```python
from build123d import *

# Parameters (mm, degrees)
SALIENTE_EXTRUIR1_DEPTH = 5


with BuildPart() as part:
    # Croquis1 → Saliente-Extruir1 (new, symmetric)
    with BuildSketch(Plane(origin=(0, 0, 0), x_dir=(-1, 0, 0), z_dir=(0, 1, 0))):
        with BuildLine():
            Line((34.242733527, 21.931170499), (171.411434738, 32.390487311))
            ThreePointArc((171.411434738, 32.390487311), (200.969948773, 5.053051121), (171.517245245, -22.398350016))
            Line((171.517245245, -22.398350016), (-0.718901979, -9.934021338))
            ThreePointArc((-0.718901979, -9.934021338), (-9.877207042, -1.281554151), (-3.23027027, 9.421621622))
            Line((-3.23027027, 9.421621622), (31.76972973, 21.421621622))
            ThreePointArc((31.76972973, 21.421621622), (32.99001932, 21.755079583), (34.242733527, 21.931170499))
        make_face()
        with BuildLine():
            Line((-0.574544152, -7.939237937), (171.661603072, -20.403566614))
            ThreePointArc((171.661603072, -20.403566614), (198.969952502, 5.049188644), (171.563496279, 30.396276368))
            Line((171.563496279, 30.396276368), (34.394795068, 19.936959556))
            ThreePointArc((34.394795068, 19.936959556), (33.393629898, 19.796228261), (32.418378378, 19.52972973))
            Line((32.418378378, 19.52972973), (-2.581621622, 7.52972973))
            ThreePointArc((-2.581621622, 7.52972973), (-7.893832134, -1.02421396), (-0.574544152, -7.939237937))
        make_face(mode=Mode.SUBTRACT)
    extrude(amount=SALIENTE_EXTRUIR1_DEPTH, both=True)


solid = part.part
```
Verification items for the finished model (mm, model axes). A direction names the side the tool comes from. Give positions to 0.01 mm unless a question says otherwise; leave off trailing zeros. Order: outer loops, then holes, each group sorted by start corner. A loop starts at its lowest first (then second) coordinate and runs counter-clockwise, first axis right, second up. Notation, with made-up numbers: M 33.25,65.25 L 61.25,65.25 A19 ccw 61.25,79.25 Z; hole C 62.25,18 d9. An arc over 180 degrees is marked long. Answer in a Markdown table with one row per item. Add a question column.
Item 1: Mould release check, pull along Z, two halves, no side actions. Record for faces 1 (the cylindrical face through (-200.96, 0.07, 5.69)), 2 (the flat face through (-101.867, 0.07, 27.088)), 3 (the cylindrical face through (-198.964, 0.07, 4.463)): released by +Z, released by -Z, zero draft, split by the parting line, or undercut.
Item 2: Section check C-C, the plane z = -5. Enter the section's corners in (x, y).
Item 3: Section check B-B, the plane y = 2. Enter the section's corners in (x, z), and give its area (3 significant figures).
Item 4: Scan lines: probe 1 along Z at (x, y) = (-13, 2.5); probe 2 along Z at (x, y) = (-65, 1); probe 3 along X at (y, z) = (1, 1.5). Record each from-to range of solid material in increasing order. Write a range as from..to.
Item 5: Tool access check on faces 4 (the flat face through (-14.025, 0.07, 15.338)), 5 (the flat face through (-15.163, 0.07, 13.614)). Record the directions out of +Z, -Z, +X, -X, +Y, -Y that give a thin tool (end or side, any length) a straight path to the whole face; none if there is none.
Item 6: Section check A-A, the plane x = -173.5. Enter the section's corners in (y, z).
Item 7: Gauge pin test, flat ends, axial feed: pin 1 (1 mm diameter, centred on y = 1, z = -1.5, fed in from -X); pin 2 (10 mm diameter, centred on x = -113, z = -10, fed in from +Y). Record the tip position at first contact, or that the pin passes through.
Filled sheet:
| question | item | result |
|---|---|---|
| 1 | face 1 | split by the parting line |
| 1 | face 2 | released by +Z |
| 1 | face 3 | undercut |
| 2 | outline | M -199.09,-5 L -196.92,-5 L -196.92,5 L -199.09,5 Z; M 6.19,-5 L 8.61,-5 L 8.61,5 L 6.19,5 Z |
| 3 | outline | M -171.52,-22.4 L 0.72,-9.93 A9.96 ccw 3.23,9.42 L -31.77,21.42 A9.96 ccw -34.24,21.93 L -171.41,32.39 A27.47 ccw long Z; hole M -171.66,-20.4 L 0.57,-7.94 A7.96 ccw 2.58,7.53 L -32.42,19.53 A7.96 ccw -34.39,19.94 L -171.56,30.4 A25.47 ccw long Z |
| 3 | area | 922 mm^2 |
| 4 | probe 1 | z = -10.93..-8.92, 12.87..14.99 |
| 4 | probe 2 | z = -14.69..-12.68, 22.27..24.28 |
| 4 | probe 3 | x = -200.75..-198.73, 7.82..9.85 |
| 5 | face 4 | +Z, +X, +Y, -Y |
| 5 | face 5 | +Y, -Y |
| 6 | outline | M -5,-22.47 L 5,-22.47 L 5,-20.47 L -5,-20.47 Z; M -5,30.47 L 5,30.47 L 5,32.47 L -5,32.47 Z |
| 7 | pin 1 | stops at x = -200.31 |
| 7 | pin 2 | passes through |
